Verification items for the finished model (mm, model axes). Give positions to 0.01 mm unless a question says otherwise; leave off trailing zeros. Write each loop counter-clockwise with the first axis right and the second up, starting at its lowest first coordinate (ties: lowest second). Pieces come first, ordered by that corner, then holes. Notation, with made-up numbers: (-20, 4) -> (6, 4) arc R6 cw to (6, 9) -> close; hole circle Ø6 at (-35.5, -12.75). An arc over 180 degrees is marked (long way). Write item = value, one per line.
Autodesk Inventor part; units mm, degrees
ref_plane "YZ Plane" through (0, 0, 0) normal (1, 0, 0) x (0, 1, 0)
ref_plane "XZ Plane" through (0, 0, 0) normal (0, 1, 0) x (-1, 0, 0)
ref_plane "XY Plane" through (0, 0, 0) normal (0, 0, 1) x (1, 0, 0)
sketch "Sketch1" plane through (0, 0, 0) normal (0, 0, 1) x (1, 0, 0)
  circle A0 centre (0, 24.5) radius 2.1828
  circle A1 centre (0, -24.5) radius 2.1828
  line L0 (6.35, -30.85) -> (-6.35, -30.85)
  line L1 (-6.35, -30.85) -> (-6.35, 30.85)
  line L2 (-6.35, 30.85) -> (6.35, 30.85)
  line L3 (6.35, 30.85) -> (6.35, -30.85)
  line L4 (6.35, -30.85) -> (-6.35, 30.85) construction
  line L5 (-6.35, -30.85) -> (6.35, 30.85) construction
  point P0 (0, 0)
  dimension "d0" = 4.3656
  dimension "d1" = 4.3656
  dimension "d2" = 49
  dimension "d3" = 24.5
  dimension "d4" = 24.5
  dimension "d5" = 12.7
  dimension "d6" = 6.35
  dimension "d7" = 6.35
extrude "Extrusion1" add sketch "Sketch1" along normal blind 1.5875
fillet "Fillet1" radius 0.7937 4 edges at (6.35, 0, 1.5875) (6.35, 0, 0) (-6.35, 0, 0) (-6.35, 0, 1.5875)
properties part number "Part I"
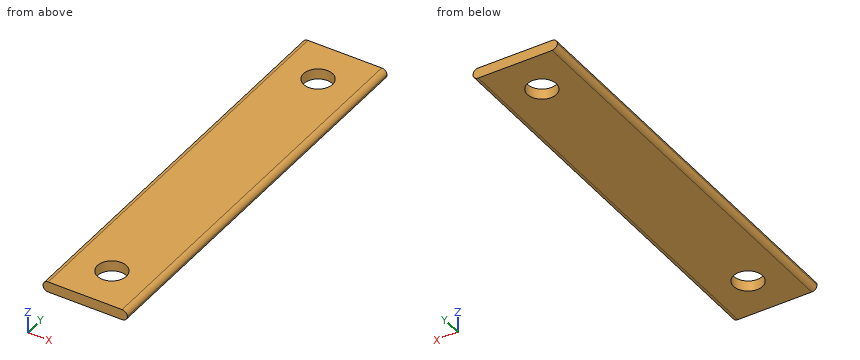
Item 1: Sectioned sample at C-C on z = 1.05. Record the cut outline in (x, y).
Response values:
outline = (-6.31, -30.85) -> (6.31, -30.85) -> (6.31, 30.85) -> (-6.31, 30.85) -> close; hole circle Ø4.37 at (0, -24.5); hole circle Ø4.37 at (0, 24.5)
Item 2: Sectioned sample at A-A on x = 0. Record the cut outline in (y, z).
Response values:
outline = (-30.85, 0) -> (-26.68, 0) -> (-26.68, 1.59) -> (-30.85, 1.59) -> close; (-22.32, 0) -> (22.32, 0) -> (22.32, 1.59) -> (-22.32, 1.59) -> close; (26.68, 0) -> (30.85, 0) -> (30.85, 1.59) -> (26.68, 1.59) -> close
Item 3: Material ranges on line 1 (Y direction, x = 0, z = 1.1); line 2 (Y direction, x = 1.25, z = 0.95); line 3 (X direction, y = 23, z = 0.45), recorded low to high.
Response values:
line_1 = -30.85 to -26.68, -22.32 to 22.32, 26.68 to 30.85
line_2 = -30.85 to -26.29, -22.71 to 22.71, 26.29 to 30.85
line_3 = -6.27 to -1.59, 1.59 to 6.27
Item 4: Go/stop test with a flat-tipped pin: P1, Ø2, axis at x = -0.5, y = 18, coming from the -Z side. Record where the tip stops, or that it passes through.
Response values:
P1 = 0
